Work out the finished part from the listing and answer in its coordinate system (mm). A direction names the side the tool comes from. Round coordinates to 2 decimals unless told otherwise and drop trailing zeros. Order: outer loops, then holes, each group sorted by start corner. A loop starts at its lowest first (then second) coordinate and runs counter-clockwise, first axis right, second up. Notation, with made-up numbers: (70.5, -37) - (122.5, -37) arc R28 ccw to (122.5, -14) - close; hole circle Ø3 at (-18.75, -35.75). An arc over 180 degrees is marked (long way). Use one line per item in the form item = value. Start each with the question number.
Q1. For a pull along Y with two mould halves and no side action, classify faces 1 (the cylindrical face through (-2.462, 10.774, 1.521)), 2 (the flat face through (-23, 0, 1)), 3 (the flat face through (-22, 13, -3.5)) as +Y half, -Y half, draft (parallel to the pull), parting line (faces both ways), or undercut.
Q2. The part is cut by section C-C on z = 0.75. State how many separate pieces and enclosed holes the cut face has, plus the area to 3 significant figures.
Q3. Find the intervals of material crossed by line 1 (X direction, y = 15.5, z = -0.75); line 2 (Y direction, x = -29.5, z = -0.75); line 3 (Z direction, x = -40, y = 22.25), in increasing order. Write a range as [from, to].
Q4. The part is cut by section B-B on z = -2.25. Determine the outline of the cut face in (x, y).
Q5. The part is cut by section D-D on x = -39.5. Determine the outline of the cut face in (y, z).
Q6. The part is cut by section A-A on x = -7.5. Determine the outline of the cut face in (y, z), plus the area to 3 significant figures.
Q7. Given P1, Ø1, axis at x = -14, z = -1, coming from the +Y side; P2, Ø1.6, axis at y = 9.5, z = -1, coming from the -X side; P3, Ø3.5, axis at y = 9.5, z = -2.5, coming from the +X side, each flat-ended and moving along its own axis, determine where each tip first touches the part or whether it passes through.
Q8. Which of the six approach directions +Z, -Z, +X, -X, +Y, -Y give full straight-line access (tool end or side, diameter ignored) to faces 4 (the flat face through (-22, 24.171, -2)), 5 (the cylindrical face through (-41.837, 12.211, 1.521)), 6 (the flat face through (-23, 13, 3)), 7 (the flat face through (-37.788, 13, -2)), 8 (the flat face through (-22, 2.171, -2))?
from build123d import *

# Parameters (mm, degrees)
SKETCH1_W               = 45
SKETCH1_H               = 25
BOSS_EXTRUDE1_DEPTH     = 3
SKETCH2_W               = 32
SKETCH2_H               = 22
BOSS_EXTRUDE2_DEPTH     = 3.5
FILLET2_R               = 0.3
FILLET3_R               = 0.3
FILLET4_R               = 0.3
FILLET5_R               = 0.3
CUT_EXTRUDE4_DEPTH      = 52.596996037
CUT_EXTRUDE4_DEPTH_BACK = 7.5
SKETCH3_R               = 1


with BuildPart() as part:
    # Sketch1 → Boss-Extrude1 (new body)
    with BuildSketch(Plane.XY):
        with Locations((-22.5, 12.5)):
            Rectangle(SKETCH1_W, SKETCH1_H)
    extrude(amount=BOSS_EXTRUDE1_DEPTH)

    # Sketch2 → Boss-Extrude2 (add)
    with BuildSketch(Plane.XY):
        with Locations((-21.788087931, 13.170864642)):
            Rectangle(SKETCH2_W, SKETCH2_H)
    extrude(amount=-BOSS_EXTRUDE2_DEPTH)

    # Fillet2
    fillet2_edges = [part.edges().sort_by_distance(p)[0] for p in [
        (-5.788087931, 2.170864642, -1.75),
    ]]
    fillet(fillet2_edges, radius=FILLET2_R)

    # Fillet3
    fillet3_edges = [part.edges().sort_by_distance(p)[0] for p in [
        (-5.788087931, 13.320864642, -3.5),
        (-21.938087931, 2.170864642, -3.5),
        (-5.875955896, 2.258732607, -3.5),
    ]]
    fillet(fillet3_edges, radius=FILLET3_R)

    # Fillet4
    fillet4_edges = [part.edges().sort_by_distance(p)[0] for p in [
        (-37.788087931, 13.320864642, -3.5),
        (-37.788087931, 2.170864642, -1.6),
        (-37.788087931, 2.258732607, -3.412132034),
    ]]
    fillet(fillet4_edges, radius=FILLET4_R)

    # Fillet5
    fillet5_edges = [part.edges().sort_by_distance(p)[0] for p in [
        (-21.788087931, 24.170864642, -3.5),
        (-5.788087931, 24.170864642, -1.6),
        (-5.875955896, 24.170864642, -3.412132034),
        (-37.788087931, 24.170864642, -1.6),
        (-37.700219965, 24.170864642, -3.412132034),
    ]]
    fillet(fillet5_edges, radius=FILLET5_R)

    # Sketch3 → Cut-Extrude4 (cut, two sides: drawn at the far end of the back side and taken through both)
    with BuildSketch(Plane(origin=(0, 0, 0), x_dir=(-1, 0, 0), z_dir=(0, 0, -1)).offset(-CUT_EXTRUDE4_DEPTH_BACK)):
        with Locations(Location((41.126309662, 21.886420327, 0), (0, 0, 180))):
            Circle(SKETCH3_R)
        with Locations(Location((2.955391169, 21.886420327, 0), (0, 0, 180))):
            Circle(SKETCH3_R)
        with Locations(Location((41.117621493, 18.886432907, 0), (0, 0, 180))):
            Circle(SKETCH3_R)
        with Locations(Location((41.108933323, 15.886445488, 0), (0, 0, 180))):
            Circle(SKETCH3_R)
        with Locations(Location((41.100245154, 12.886458069, 0), (0, 0, 180))):
            Circle(SKETCH3_R)
        with Locations(Location((2.947370185, 18.886431049, 0), (0, 0, 180))):
            Circle(SKETCH3_R)
        with Locations(Location((2.939349201, 15.886441772, 0), (0, 0, 180))):
            Circle(SKETCH3_R)
        with Locations(Location((2.931328218, 12.886452495, 0), (0, 0, 180))):
            Circle(SKETCH3_R)
        with Locations(Location((2.923307234, 9.886463217, 0), (0, 0, 180))):
            Circle(SKETCH3_R)
        with Locations(Location((2.91528625, 6.88647394, 0), (0, 0, 180))):
            Circle(SKETCH3_R)
    extrude(amount=CUT_EXTRUDE4_DEPTH + CUT_EXTRUDE4_DEPTH_BACK, mode=Mode.SUBTRACT)


solid = part.part
Found:
q1.face_1 = undercut
q1.face_2 = -Y half
q1.face_3 = draft
q2.separate_pieces = 1
q2.enclosed_holes = 10
q2.area = 1,090 mm²
q3.line_1 = [-37.79, -5.79]
q3.line_2 = [2.17, 24.17]
q3.line_3 = [0, 3]
q4.outline = (-37.79, 2.47) arc R0.3 ccw to (-37.49, 2.17) - (-6.09, 2.17) arc R0.3 ccw to (-5.79, 2.47) - (-5.79, 23.87) arc R0.3 ccw to (-6.09, 24.17) - (-37.49, 24.17) arc R0.3 ccw to (-37.79, 23.87) - close
q5.outline = (0, 0) - (25, 0) - (25, 3) - (0, 3) - close
q6.outline = (0, 0) - (2.17, 0) - (2.17, -3.2) arc R0.3 ccw to (2.47, -3.5) - (23.87, -3.5) arc R0.3 ccw to (24.17, -3.2) - (24.17, 0) - (25, 0) - (25, 3) - (0, 3) - close
q6.area = 152 mm²
q7.P1 = 24.17
q7.P2 = -37.79
q7.P3 = -5.79
q8.face_4 = -Z, +X, -X, +Y
q8.face_5 = +Z, -Z
q8.face_6 = +Z, +X, -X, +Y, -Y
q8.face_7 = -Z, -X, +Y, -Y
q8.face_8 = -Z, +X, -X, -Y
